Model file for the job. Use its own axes, mm. Face numbers are marked on the shaded views. A direction names the side the tool comes from. Round coordinates to 2 decimals unless told otherwise and drop trailing zeros. Order: outer loops, then holes, each group sorted by start corner. A loop starts at its lowest first (then second) coordinate and runs counter-clockwise, first axis right, second up. Notation, with made-up numbers: (-39.5, 55.25) -> (-7.5, 55.25) arc R27 ccw to (-7.5, 77.25) -> close; hole circle Ø9 at (77, 21). An arc over 180 degrees is marked (long way). Answer as CSV lines item,"result".
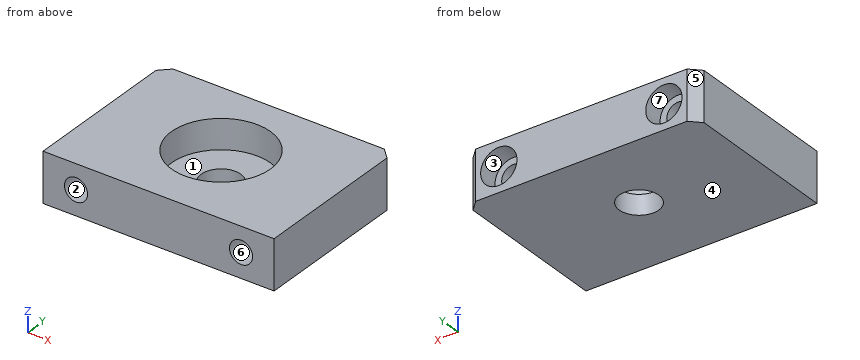
```python
from build123d import *

# Parameters (mm, degrees)
SKETCH_1_W                   = 70
SKETCH_1_H                   = 50
EXTRUDE_1_DEPTH              = 15
SKETCH_2_R                   = 6
CUT_EXTRUDE_1_DEPTH          = 88.321245983
CHAMFER_1_SIZE               = 3
HOLE_WIZARD_M6_1_D           = 7
HOLE_WIZARD_M6_1_CBORE_D     = 11
HOLE_WIZARD_M6_1_CBORE_DEPTH = 6
SKETCH_5_R                   = 15
CUT_EXTRUDE_2_DEPTH          = 9


with BuildPart() as part:
    # 草图1 → 凸台-拉伸1 (new body)
    with BuildSketch(Plane.XY):
        with Locations((35, 25)):
            Rectangle(SKETCH_1_W, SKETCH_1_H)
    extrude(amount=EXTRUDE_1_DEPTH)

    # 草图2 → 切除-拉伸1 (cut, through all)
    with BuildSketch(Plane.XY.offset(15)):
        with Locations((35, 26)):
            Circle(SKETCH_2_R)
    extrude(amount=-CUT_EXTRUDE_1_DEPTH, mode=Mode.SUBTRACT)

    # 倒角1
    chamfer_1_edges = [part.edges().sort_by_distance(p)[0] for p in [
        (0, 50, 7.5),
        (70, 50, 7.5),
    ]]
    chamfer(chamfer_1_edges, length=CHAMFER_1_SIZE)

    # M6 六角凹头螺钉的柱形沉头孔1 (through all)
    with Locations(Plane(origin=(0, 50, 0), x_dir=(-1, 0, 0), z_dir=(0, 1, 0))):
        with Locations((-10, 7.5), (-60, 7.5)):
            CounterBoreHole(HOLE_WIZARD_M6_1_D / 2, HOLE_WIZARD_M6_1_CBORE_D / 2, HOLE_WIZARD_M6_1_CBORE_DEPTH)

    # 草图5 → 切除-拉伸2 (cut)
    with BuildSketch(Plane.XY.offset(15)):
        with Locations((35, 26)):
            Circle(SKETCH_5_R)
    extrude(amount=-CUT_EXTRUDE_2_DEPTH, mode=Mode.SUBTRACT)


solid = part.part
```
Q1. Saw through at A-A (z = 7.5). Write the cut outline in (x, y).
Checks:
outline,"(0, 0) -> (6.5, 0) -> (6.5, 44) -> (4.5, 44) -> (4.5, 50) -> (3, 50) -> (0, 47) -> close; (13.5, 0) -> (56.5, 0) -> (56.5, 44) -> (54.5, 44) -> (54.5, 50) -> (15.5, 50) -> (15.5, 44) -> (13.5, 44) -> close; (63.5, 0) -> (70, 0) -> (70, 47) -> (67, 50) -> (65.5, 50) -> (65.5, 44) -> (63.5, 44) -> close; hole circle Ø30 at (35, 26)"
Q2. Saw through at D-D (z = 14.25). Write the cut outline in (x, y).
Checks:
outline,"(0, 0) -> (70, 0) -> (70, 47) -> (67, 50) -> (3, 50) -> (0, 47) -> close; hole circle Ø30 at (35, 26)"
Q3. Wall check: L1, parallel to X at y = 9.5, z = 10; L2, parallel to Z at x = 10, y = 45.9; L3, parallel to Z at x = 60, y = 9. Give the ranges that are in metal, low to high. Write a range as [from, to].
Checks:
L1,"[0, 7.55], [12.45, 57.55], [62.45, 70]"
L2,"[0, 2], [13, 15]"
L3,"[0, 4], [11, 15]"
Q4. Saw through at B-B (y = 26). Write the cut outline in (x, z).
Checks:
outline,"(0, 0) -> (29, 0) -> (29, 6) -> (20, 6) -> (20, 15) -> (0, 15) -> close; (41, 0) -> (70, 0) -> (70, 15) -> (50, 15) -> (50, 6) -> (41, 6) -> close; hole circle Ø7 at (10, 7.5); hole circle Ø7 at (60, 7.5)"
Q5. Mould opens along X. For the marked faces 4, 5, 6 and 7 say: +X half, -X half, draft (parallel to the pull), parting line (faces both ways), or undercut.
Checks:
face 4,"draft"
face 5,"-X half"
face 6,"undercut"
face 7,"undercut"
Q6. Flat gauge pins, fed straight in: pin 1 (5.5 mm diameter, centred on x = 9.5, z = 9, fed in from +Y); pin 2 (15 mm diameter, centred on x = 38.5, y = 20.5, fed in from +Z). Where does each tip first touch, or does it go through?
Checks:
pin 1,"y = 44"
pin 2,"z = 6"
Q7. Tool access for the marked faces 1, 2 and 3: list every direction of +Z, -Z, +X, -X, +Y, -Y with a clear straight run to the whole face (end or side of a thin tool).
Checks:
face 1,"+Z"
face 2,"+Y, -Y"
face 3,"+Y"
Q8. Saw through at C-C (x = 10). Write the cut outline in (y, z), plus the area to 3 significant figures.
Checks:
outline,"(0, 0) -> (50, 0) -> (50, 2) -> (44, 2) -> (44, 4) -> (0, 4) -> close; (0, 11) -> (44, 11) -> (44, 13) -> (50, 13) -> (50, 15) -> (0, 15) -> close"
area,"376 mm²"
